```python
from build123d import *

# Parameters (mm, degrees)
CROQUIS1_W                                           = 50
CROQUIS1_H                                           = 50
CROQUIS1_R                                           = 2
SALIENTE_EXTRUIR2_DEPTH                              = 12
CROQUIS4_W                                           = 3.2
CROQUIS4_H                                           = 40
SALIENTE_EXTRUIR5_DEPTH                              = 10.2
CORTAR_EXTRUIR2_START                                = -50
CROQUIS7_R                                           = 2
CORTAR_EXTRUIR2_DEPTH                                = 50
REFRENTADO_PARA_TORNILLO_TAP_N_CON_CABEZ_D           = 4.5
REFRENTADO_PARA_TORNILLO_TAP_N_CON_CABEZ_CSINK_D     = 8.96
REFRENTADO_PARA_TORNILLO_TAP_N_CON_CABEZ_CSINK_ANGLE = 90
SALIENTE_EXTRUIR14_DEPTH                             = 10.05
SALIENTE_EXTRUIR15_START                             = 2.95
SALIENTE_EXTRUIR15_DEPTH                             = 1.95
SALIENTE_EXTRUIR16_START                             = 10.05
SALIENTE_EXTRUIR16_DEPTH                             = 1.95


with BuildPart() as part:
    # Croquis1 → Saliente-Extruir2 (new body)
    with BuildSketch(Plane.XY):
        Rectangle(CROQUIS1_W, CROQUIS1_H)
        Circle(CROQUIS1_R, mode=Mode.SUBTRACT)
    extrude(amount=SALIENTE_EXTRUIR2_DEPTH)

    # Croquis2 → Cortar-Revolución1 (revolve, cut)
    with BuildSketch(Plane(origin=(0, 0, 0), x_dir=(0, 0, -1), z_dir=(1, 0, 0))):
        Polygon((-12, 15.2), (-12, 0), (-1.8, 0), (-1.8, 10), (-9.8, 15.2), align=None)
    revolve(axis=Axis((0, 0, 12), (0, 0, -1)), mode=Mode.SUBTRACT)

    # Croquis4 → Saliente-Extruir5 (add)
    with BuildSketch(Plane.XY.offset(12)):
        with Locations((-6.6, 0)):
            Rectangle(CROQUIS4_W, CROQUIS4_H)
        with Locations((6.6, 0)):
            Rectangle(CROQUIS4_W, CROQUIS4_H)
    extrude(amount=-SALIENTE_EXTRUIR5_DEPTH)

    # Croquis7 → Cortar-Extruir2 (cut)
    with BuildSketch(Plane.ZY.offset(25).offset(CORTAR_EXTRUIR2_START)):
        with Locations((7, 0)):
            Circle(CROQUIS7_R)
    extrude(amount=CORTAR_EXTRUIR2_DEPTH, mode=Mode.SUBTRACT)

    # Refrentado para tornillo tap_n con cabez (through all)
    with Locations(Plane.ZY.offset(25)):
        with Locations((7, 0)):
            CounterSinkHole(REFRENTADO_PARA_TORNILLO_TAP_N_CON_CABEZ_D / 2, REFRENTADO_PARA_TORNILLO_TAP_N_CON_CABEZ_CSINK_D / 2, counter_sink_angle=REFRENTADO_PARA_TORNILLO_TAP_N_CON_CABEZ_CSINK_ANGLE)

    # Croquis17 → Refrentado para tornillo tap_n con c 2 (revolve, cut)
    with BuildSketch(Plane(origin=(0, 0, 1.8), x_dir=(0, -1, 0), z_dir=(1, 0, 0))):
        Polygon((0, 0), (0, 1.8), (2.25, 1.8), (2.25, 2.23), (4.48, 0), align=None)
    revolve(axis=Axis((0, 0, 8.15), (0, 0, -1)), mode=Mode.SUBTRACT)

    # Croquis19 → Saliente-Extruir14 (add)
    with BuildSketch(Plane.ZY.offset(25)):
        Polygon((12, 45), (10, 43), (10, 25), (0, 25), (0, 23.05), (10, 23.05), (12, 23.05), (12, 25), align=None)
    extrude(amount=SALIENTE_EXTRUIR14_DEPTH)

    # Croquis12 → Saliente-Extruir15 (add)
    with BuildSketch(Plane.ZY.offset(25).offset(SALIENTE_EXTRUIR15_START)):
        Polygon((12, 45), (-8, 25), (12, 25), align=None)
    extrude(amount=SALIENTE_EXTRUIR15_DEPTH)

    # Croquis12<3> → Saliente-Extruir16 (add)
    with BuildSketch(Plane.ZY.offset(25).offset(SALIENTE_EXTRUIR16_START)):
        Polygon((12, 45), (-8, 25), (12, 25), align=None)
    extrude(amount=-SALIENTE_EXTRUIR16_DEPTH)


solid = part.part
```
Geometry check sheet. Reference: the model listing, model coordinates, mm. A direction names the side the tool comes from. Give positions to 0.01 mm unless a question says otherwise; leave off trailing zeros. Order: outer loops, then holes, each group sorted by start corner. A loop starts at its lowest first (then second) coordinate and runs counter-clockwise, first axis right, second up. Notation, with made-up numbers: (38.5, -40) -> (48.5, -40) arc R33 ccw to (48.5, -8) -> close; hole circle Ø11 at (63, -13). An arc over 180 degrees is marked (long way). Write each question's results on one line, items separated by ' | '. Start each with the question number.
(1) Sectioned sample at A-A (x = 0). Enter the section's corners in (y, z).
(2) Sectioned sample at B-B (x = 17.5). Enter the section's corners in (y, z), plus the area to 3 significant figures.
(3) Sectioned sample at D-D (y = 0). Give the number of separate pieces and of enclosed holes in the cut face, plus the area to 3 significant figures.
(4) Scan lines: line 1 (Y direction, x = 6.1, z = 7); line 2 (X direction, y = 8.5, z = 6.5); line 3 (X direction, y = 28.5, z = 2.75). Record each from-to range of solid material in increasing order.
(5) Sectioned sample at C-C (y = -19.5). Enter the section's corners in (x, z).
(6) Mould release check, pull along X, two halves, no side actions. Record for faces 1 (the face through (-11.48, -0.16, 4.08)), 2 (the face through (-22.88, 0.71, 4.75)), 3 (the face through (-1, 25, 6)): pulls with the +X half, pulls with the -X half, needs draft (parallel to the pull), parting line crosses it, or undercut.
(7) Gauge pin test, flat ends, axial feed: P1, Ø2.5, axis at x = -27, y = 32, coming from the -Z side; P2, Ø1.5, axis at y = 18.5, z = 7.5, coming from the -X side; P3, Ø0.6, axis at x = -34.5, z = -3, coming from the -Y side. Record the tip position at first contact, or that the pin passes through.
(8) Access from +Z, -Z, +X, -X, +Y, -Y to the whole of each face (thin tool, end or side, straight path). Record for faces 4 (the face through (-18.474, 0.676, 4.854)), 5 (the face through (-9, 0, 1.8)), 6 (the face through (-29, 25, -4)), 7 (the face through (-25, 35, 11)), 8 (the face through (-31, 34, 10)).
Answer below:
1) outline: (-25, 0) -> (-2.68, 0) -> (-4.48, 1.8) -> (-10, 1.8) -> (-15.2, 9.8) -> (-15.2, 12) -> (-25, 12) -> close; (2.68, 0) -> (25, 0) -> (25, 12) -> (15.2, 12) -> (15.2, 9.8) -> (10, 1.8) -> (4.48, 1.8) -> close
2) outline: (-25, 0) -> (25, 0) -> (25, 12) -> (-25, 12) -> close; hole circle Ø4.5 at (0, 7) | area: 584 mm2
3) separate pieces: 6 | enclosed holes: 0 | area: 246 mm2
4) line 1: -25 to -2.25, 2.25 to 25 | line 2: -25 to -9.91, -8.2 to -5, 5 to 8.2, 9.91 to 25 | line 3: -35.05 to -33.1, -29.9 to -27.95
5) outline: (-25, 0) -> (25, 0) -> (25, 12) -> (-25, 12) -> close
6) face 1: undercut | face 2: pulls with the -X half | face 3: needs draft
7) P1: z = -1.81 | P2: x = -25 | P3: y = 25
8) face 4: +X, -X | face 5: +Z | face 6: -Z, +X, -X, -Y | face 7: +Z, -Z, +X, +Y | face 8: -Z, +Y
